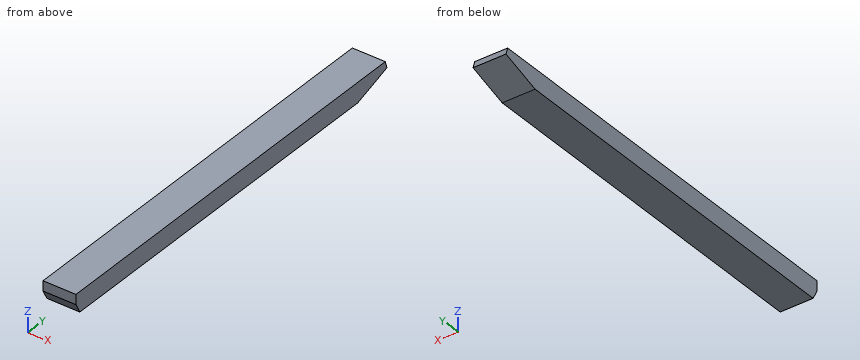
from build123d import *

# Parameters (mm, degrees)
ESQUISSE1_W             = 63
ESQUISSE1_H             = 800
BOSS_EXTRU_1_DEPTH      = 38
ENL_V_MAT_EXTRU_1_DEPTH = 804.376001633
ENL_V_MAT_EXTRU_2_DEPTH = 804.376001633


with BuildPart() as part:
    # Esquisse1 → Boss.-Extru.1 (new body)
    with BuildSketch(Plane.XY):
        with Locations((31.5, 400)):
            Rectangle(ESQUISSE1_W, ESQUISSE1_H)
    extrude(amount=BOSS_EXTRU_1_DEPTH)

    # Esquisse2 → Enlèv. mat.-Extru.1 (cut, through all)
    with BuildSketch(Plane.ZY):
        Polygon((24.368977217, 800), (0, 725), (0, 800), align=None)
        Polygon((19, 0), (0, 10), (0, 0), align=None)
    extrude(amount=-ENL_V_MAT_EXTRU_1_DEPTH, mode=Mode.SUBTRACT)

    # Esquisse3 → Enlèv. mat.-Extru.2 (cut, through all)
    with BuildSketch(Plane.ZY):
        Polygon((24.368977217, 800), (38, 795.571012218), (38, 800), align=None)
    extrude(amount=-ENL_V_MAT_EXTRU_2_DEPTH, mode=Mode.SUBTRACT)


solid = part.part
Input: part model. Units: mm. Frame: model coordinates. Round coordinates to 2 decimals unless told otherwise and drop trailing zeros. Order: outer loops, then holes, each group sorted by start corner. A loop starts at its lowest first (then second) coordinate and runs counter-clockwise, first axis right, second up. Notation, with made-up numbers: (-10, 36.5) - (20, 36.5) arc R20 ccw to (20, 47.5) - close; hole circle Ø9 at (1.25, 15). An arc over 180 degrees is marked (long way). Answer as a JSON object with one key per item and string values. Group by question number.
(1) Material intervals for probe 1 along Y at (x, z) = (48, 29); probe 2 along Y at (x, z) = (55.5, 30); probe 3 along Z at (x, y) = (7.5, 736.5), sorted ascending. Write a range as from..to.
(2) Cut plane B-B (z = 11). Return loops of the section in (x, y), then the cut area to 3 significant figures.
(3) Cut plane A-A (x = 25). Return loops of the section in (y, z), then the cut area to 3 significant figures.
Here are the results:
{
 "1": {"probe 1": "y = 0..798.5", "probe 2": "y = 0..798.17", "probe 3": "z = 3.74..38"},
 "2": {"outline": "(0, 4.21) - (63, 4.21) - (63, 758.85) - (0, 758.85) - close", "area": "47,500 mm^2"},
 "3": {"outline": "(0, 19) - (10, 0) - (725, 0) - (800, 24.37) - (795.57, 38) - (0, 38) - close", "area": "29,400 mm^2"}
}
